from build123d import *

# Parameters (mm, degrees)
F0_R     = 11
F1_DEPTH = 3.5
F2_R     = 5
F3_SIZE  = 1


with BuildPart() as f1:
    # F0 (on Top) → F1 (new body, symmetric)
    with BuildSketch(Plane.XY):
        with BuildLine():
            Line((17.023025, 33.009872), (0, 45))
            Line((0, 45), (-17.023025, 33.009872))
            Line((-17.023025, 33.009872), (-9.861474, 11.302714))
            ThreePointArc((-9.861474, 11.302714), (0, 15), (9.861474, 11.302714))
            Line((9.861474, 11.302714), (17.023025, 33.009872))
        make_face()
        with Locations((0, 27.524821)):
            Circle(F0_R, mode=Mode.SUBTRACT)
        with BuildLine():
            ThreePointArc((-4.8577, -14.191644), (-12.990381, -7.5), (-14.719174, 2.88893))
            Line((-14.719174, 2.88893), (-37.0989, -1.762564))
            Line((-37.0989, -1.762564), (-38.971143, -22.5))
            Line((-38.971143, -22.5), (-20.075875, -31.247308))
            Line((-20.075875, -31.247308), (-4.8577, -14.191644))
        make_face()
        with Locations((-23.837195, -13.762411)):
            Circle(F0_R, mode=Mode.SUBTRACT)
        with BuildLine():
            Line((37.0989, -1.762564), (14.719174, 2.88893))
            ThreePointArc((14.719174, 2.88893), (14.929628, 1.451273), (15, 0))
            ThreePointArc((15, 0), (12.203801, -8.721654), (4.8577, -14.191644))
            Line((4.8577, -14.191644), (20.075875, -31.247308))
            Line((20.075875, -31.247308), (38.971143, -22.5))
            Line((38.971143, -22.5), (37.0989, -1.762564))
        make_face()
        with Locations((23.837195, -13.762411)):
            Circle(F0_R, mode=Mode.SUBTRACT)
        with BuildLine():
            ThreePointArc((9.861474, 11.302714), (0, 15), (-9.861474, 11.302714))
            ThreePointArc((-9.861474, 11.302714), (-12.990381, 7.5), (-14.719174, 2.88893))
            ThreePointArc((-14.719174, 2.88893), (-12.990381, -7.5), (-4.8577, -14.191644))
            ThreePointArc((-4.8577, -14.191644), (0, -15), (4.8577, -14.191644))
            ThreePointArc((4.8577, -14.191644), (12.203801, -8.721654), (15, 0))
            ThreePointArc((15, 0), (14.929628, 1.451273), (14.719174, 2.88893))
            ThreePointArc((14.719174, 2.88893), (12.990381, 7.5), (9.861474, 11.302714))
        make_face()
        Circle(F0_R, mode=Mode.SUBTRACT)
    extrude(amount=F1_DEPTH, both=True)

    # F2
    f2_edges = [f1.edges().sort_by_distance(p)[0] for p in [
        (17.023025, 33.009872, 0),
        (9.861474, 11.302714, 0),
        (14.719174, 2.88893, 0),
        (37.0989, -1.762564, 0),
        (38.971143, -22.5, 0),
        (4.8577, -14.191644, 0),
        (20.075875, -31.247308, 0),
        (-4.8577, -14.191644, 0),
        (-20.075875, -31.247308, 0),
        (-38.971143, -22.5, 0),
        (-37.0989, -1.762564, 0),
        (-14.719174, 2.88893, 0),
        (-9.861474, 11.302714, 0),
        (-17.023025, 33.009872, 0),
        (0, 45, 0),
    ]]
    fillet(f2_edges, radius=F2_R)

    # F3
    f3_edges = [f1.edges().sort_by_distance(p)[0] for p in [
        (8.435968, 39.058145, -3.5),
        (-38.04333, -12.22331, 3.5),
    ]]
    chamfer(f3_edges, length=F3_SIZE)


solid = f1.part
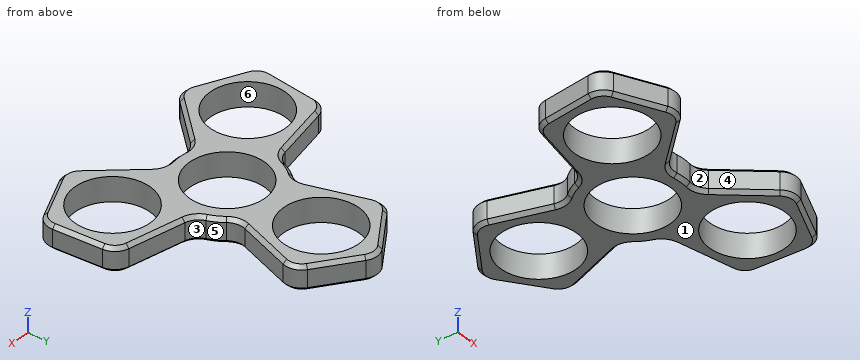
Verification items for the finished model (mm, model axes). Face numbers are marked on the shaded views. A direction names the side the tool comes from. Give positions to 0.01 mm unless a question says otherwise; leave off trailing zeros. Order: outer loops, then holes, each group sorted by start corner. A loop starts at its lowest first (then second) coordinate and runs counter-clockwise, first axis right, second up. Notation, with made-up numbers: M -9,66 L 43,66 A34 ccw 43,101 Z; hole C 58,49.25 d5. An arc over 180 degrees is marked long. Answer as a JSON object with one key per item and string values. Group by question number.
1) Cross-section at C-C (y = 37.5). Enter the section's corners in (x, z).
2) Cross-section at B-B (x = -28). Enter the section's corners in (y, z).
3) Access from +Z, -Z, +X, -X, +Y, -Y to the whole of each face (thin tool, end or side, straight path). Record for the marked faces 4, 5 and 6.
4) Depth check by flat-ended pin: pin 1 Ø1.5 at (x, z) = (2.5, -1.5) entering from +Y; pin 2 Ø1 at (y, z) = (36, -0.5) entering from +X; pin 3 Ø2 at (y, z) = (36, -1) entering from -X. Enter the tip coordinate at first touch or a pass-through.
5) Mould release check, pull along Y, two halves, no side actions. Record for the marked faces 1, 2 and 3: released by +Y, released by -Y, zero draft, split by the parting line, or undercut.
6) Cross-section at A-A (x = 0). Enter the section's corners in (y, z).
7) Cross-section at D-D (z = -1). Give the number of separate pieces and of enclosed holes in the cut face, then the cut area to 3 significant figures.
8) Scan lines: line 1 along Y through (x, z) = (0, -0.25); line 2 along Y through (x, z) = (-7, 0); line 3 along X through (y, z) = (-8.5, -2). Record each from-to range of solid material in increasing order. Write a range as [from, to].
Result sheet:
{
 "1": {"outline": "M -10.65,-2.5 L -8.91,-3.5 L -4.64,-3.5 L -4.64,3.5 L -8.91,3.5 L -10.65,2.5 Z; M 4.64,-3.5 L 8.91,-3.5 L 10.65,-2.5 L 10.65,2.5 L 8.91,3.5 L 4.64,3.5 Z"},
 "2": {"outline": "M -27.58,-2.5 L -26.48,-3.5 L -23.94,-3.5 L -23.94,3.5 L -26.48,3.5 L -27.58,2.5 Z; M -3.58,-3.5 L -0.89,-3.5 L 0.13,-2.5 L 0.13,2.5 L -0.89,3.5 L -3.58,3.5 Z"},
 "3": {"face 4": "+Z, -Z, -Y", "face 5": "+Z, -Z, +X", "face 6": "+Z, -Z"},
 "4": {"pin 1": "stops at y = 43.57", "pin 2": "stops at x = 13.49", "pin 3": "stops at x = -14.19"},
 "5": {"face 1": "zero draft", "face 2": "released by -Y", "face 3": "undercut"},
 "6": {"outline": "M -15,-2.5 L -14,-3.5 L -11,-3.5 L -11,3.5 L -14,3.5 L -15,2.5 Z; M 11,-3.5 L 16.52,-3.5 L 16.52,3.5 L 11,3.5 Z; M 38.52,-3.5 L 42.88,-3.5 L 43.88,-2.5 L 43.88,2.5 L 42.88,3.5 L 38.52,3.5 Z"},
 "7": {"separate pieces": "1", "enclosed holes": "4", "area": "1,390 mm2"},
 "8": {"line 1": "y = [-15, -11], [11, 16.52], [38.52, 43.88]", "line 2": "y = [-16.59, -8.49], [8.49, 19.04], [36.01, 40.07]", "line 3": "x = [-37.71, -33.5], [-14.18, -6.98], [6.98, 14.18], [33.5, 37.71]"}
}
